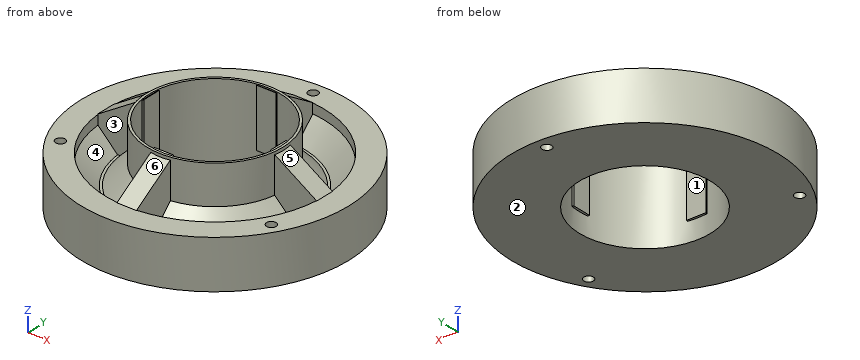
```python
from build123d import *

# Parameters (mm, degrees)
SKETCH_R        = 27.5
SKETCH_R_2      = 22.5
SKETCH_R_3      = 1
PAD_DEPTH       = 10
SKETCH001_R     = 22.5
SKETCH001_R_2   = 14
PAD001_DEPTH    = 4
CHAMFER_SIZE    = 4
PAD002_DEPTH    = 2
PAD003_DEPTH    = 2
SKETCH004_R     = 14
SKETCH004_R_2   = 13.5
PAD004_DEPTH    = 16
CHAMFER001_SIZE = 4


with BuildPart() as part:
    # Sketch → Pad (new body)
    with BuildSketch(Plane.XY):
        Circle(SKETCH_R)
        Circle(SKETCH_R_2, mode=Mode.SUBTRACT)
        with Locations((0, 25)):
            Circle(SKETCH_R_3, mode=Mode.SUBTRACT)
        with Locations((-21.650635, -12.5)):
            Circle(SKETCH_R_3, mode=Mode.SUBTRACT)
        with Locations((21.650635, -12.5)):
            Circle(SKETCH_R_3, mode=Mode.SUBTRACT)
    extrude(amount=PAD_DEPTH)

    # Sketch001 → Pad001 (join)
    with BuildSketch(Plane.XY):
        Circle(SKETCH001_R)
        Circle(SKETCH001_R_2, mode=Mode.SUBTRACT)
    extrude(amount=PAD001_DEPTH)

    # Chamfer
    chamfer_edges = [part.edges().sort_by_distance(p)[0] for p in [
        (-22.5, 0, 4),
    ]]
    chamfer(chamfer_edges, length=CHAMFER_SIZE)

    # Sketch002 → Pad002 (join, symmetric)
    with BuildSketch(Plane.XZ):
        Polygon((22.5, 10), (22.5, 4), (13, 4), (13, 16), align=None)
        Polygon((-22.5, 10), (-22.5, 4), (-13, 4), (-13, 16), align=None)
    extrude(amount=PAD002_DEPTH, both=True)

    # Sketch003 → Pad003 (join, symmetric)
    with BuildSketch(Plane.YZ):
        Polygon((13, 4), (22.5, 4), (22.5, 10), (13, 16), align=None)
        Polygon((-13, 4), (-22.5, 4), (-22.5, 10), (-13, 16), align=None)
    extrude(amount=PAD003_DEPTH, both=True)

    # Sketch004 → Pad004 (join)
    with BuildSketch(Plane.XY):
        Circle(SKETCH004_R)
        Circle(SKETCH004_R_2, mode=Mode.SUBTRACT)
    extrude(amount=PAD004_DEPTH)

    # Chamfer001
    chamfer001_edges = [part.edges().sort_by_distance(p)[0] for p in [
        (9.899495, 9.899495, 4),
        (9.899495, -9.899495, 4),
        (-9.899495, -9.899495, 4),
        (-9.899495, 9.899495, 4),
    ]]
    chamfer(chamfer001_edges, length=CHAMFER001_SIZE)


solid = part.part
```
Input: part model. Units: mm. Frame: model coordinates. Face numbers are marked on the shaded views. A direction names the side the tool comes from. Give positions to 0.01 mm unless a question says otherwise; leave off trailing zeros. Order: outer loops, then holes, each group sorted by start corner. A loop starts at its lowest first (then second) coordinate and runs counter-clockwise, first axis right, second up. Notation, with made-up numbers: M 74.5,40 L 97.5,40 A24 cw 97.5,52 Z; hole C 55,58.25 d5. An arc over 180 degrees is marked long. One line per question, with ' | ' between items. Start each with the question number.
1. First-contact query: pin 1 Ø1 at (x, z) = (7.5, 13.5) entering from +Y; pin 2 Ø3 at (y, z) = (16.5, 2) entering from +X; pin 3 Ø3 at (x, z) = (20.5, 10) entering from -Y. Flat tips, straight axial feed; report the tip coordinate or a pass-through.
2. Section query D-D (y = 25). Return the cut outline in (x, z), and give its area (3 significant figures).
3. Section query C-C (z = 6.75). Count the separate pieces of the cut face and the enclosed holes in it, and give its area (3 significant figures).
4. Section query B-B (x = 0). Return the cut outline in (y, z), and give its area (3 significant figures).
5. Material intervals for probe 1 along Y at (x, z) = (0, 6.5); probe 2 along Y at (x, z) = (14, 8.25); probe 3 along Z at (x, y) = (3, -24), sorted ascending. Write a range as [from, to].
6. Section query A-A (y = 0). Return the cut outline in (x, z).
7. Access query for the marked faces 1, 2 and 3. Directions: +Z, -Z, +X, -X, +Y, -Y. A direction counts if a zero-diameter tool reaches every point of the face in a straight line with its end or side. Return the directions, or none.
8. Pull-direction query (Y, two-part tool) for the marked faces 4, 5 and 6; classes: released by +Y, released by -Y, zero draft, split by the parting line, or undercut.
Here are the results:
1) pin 1: y = 12.12 | pin 2: x = 23.05 | pin 3: y = -19.88
2) outline: M -11.46,0 L -1,0 L -1,10 L -11.46,10 Z; M 1,0 L 11.46,0 L 11.46,10 L 1,10 Z | area: 209 mm²
3) separate pieces: 1 | enclosed holes: 8 | area: 1,210 mm²
4) outline: M -27.5,0 L -13.5,0 L -13.5,4 L -13,4 L -13,16 L -13.5,15.68 L -13.5,16 L -14,16 L -14,15.37 L -22.5,10 L -27.5,10 Z; M 13,4 L 13.5,4 L 13.5,0 L 24,0 L 24,10 L 22.5,10 L 14,15.37 L 14,16 L 13.5,16 L 13.5,15.68 L 13,16 Z; M 26,0 L 27.5,0 L 27.5,10 L 26,10 Z | area: 323 mm²
5) probe 1: [-27.5, -13], [13, 24], [26, 27.5] | probe 2: [-23.67, -17.61], [-2, 2], [17.61, 23.67] | probe 3: [0, 10]
6) outline: M -27.5,0 L -13.5,0 L -13.5,4 L -13,4 L -13,16 L -13.5,15.68 L -13.5,16 L -14,16 L -14,15.37 L -22.5,10 L -27.5,10 Z; M 13,4 L 13.5,4 L 13.5,0 L 27.5,0 L 27.5,10 L 22.5,10 L 14,15.37 L 14,16 L 13.5,16 L 13.5,15.68 L 13,16 Z
7) face 1: +Z, -Z | face 2: -Z, +X, -X, +Y, -Y | face 3: +Z
8) face 4: undercut | face 5: zero draft | face 6: released by -Y
